Part model, mm, in its own coordinate system. A direction names the side the tool comes from. Give positions to 0.01 mm unless a question says otherwise; leave off trailing zeros. Order: outer loops, then holes, each group sorted by start corner. A loop starts at its lowest first (then second) coordinate and runs counter-clockwise, first axis right, second up. Notation, with made-up numbers: M 32.25,19.5 L 80.25,19.5 A18 cw 80.25,53.5 Z; hole C 2.25,32 d6. An arc over 180 degrees is marked long. One line per question, with ' | ' between items.
```python
from build123d import *

# Parameters (mm, degrees)
SKETCH_1_W          = 20
SKETCH_1_H          = 20
SKETCH_1_W_2        = 16
SKETCH_1_H_2        = 16
EXTRUDE_1_DEPTH     = 970
SKETCH_2_R          = 4.05
CUT_EXTRUDE_1_DEPTH = 20
SKETCH_4_W          = 21.376287738
SKETCH_4_H          = 29.089038522
CUT_EXTRUDE_3_DEPTH = 50
SKETCH_5_R          = 2.2
CUT_EXTRUDE_4_DEPTH = 30
SKETCH_6_R          = 1
CUT_EXTRUDE_5_DEPTH = 10
M4X0_7_1_D          = 3.3
M4X0_7_1_DEPTH      = 11.5
M4X0_7_1_TIP        = 0.991420021
SKETCH_12_R         = 1
CUT_EXTRUDE_7_DEPTH = 10
M4X0_7_6_D          = 3.3
M4X0_7_6_DEPTH      = 11.5
M4X0_7_6_TIP        = 0.991420021
SKETCH_15_R         = 2.1
CUT_EXTRUDE_8_DEPTH = 21
SKETCH_16_R         = 1
CUT_EXTRUDE_9_DEPTH = 10
M4X0_7_7_D          = 3.3
M4X0_7_7_DEPTH      = 11.5
M4X0_7_7_TIP        = 0.991420021


with BuildPart() as part:
    # ｽｹｯﾁ1 → ﾎﾞｽ - 押し出し1 (new body)
    with BuildSketch(Plane.XY):
        Rectangle(SKETCH_1_W, SKETCH_1_H)
        Rectangle(SKETCH_1_W_2, SKETCH_1_H_2, mode=Mode.SUBTRACT)
    extrude(amount=EXTRUDE_1_DEPTH)

    # ｽｹｯﾁ2 → ｶｯﾄ - 押し出し1 (cut)
    with BuildSketch(Plane(origin=(10, 0, 0), x_dir=(0, 0, -1), z_dir=(1, 0, 0))):
        with Locations((-50, 0)):
            Circle(SKETCH_2_R)
    extrude(amount=-CUT_EXTRUDE_1_DEPTH, mode=Mode.SUBTRACT)

    # ｽｹｯﾁ4 → ｶｯﾄ - 押し出し3 (cut)
    with BuildSketch(Plane.XY.offset(970)):
        Rectangle(SKETCH_4_W, SKETCH_4_H)
    extrude(amount=-CUT_EXTRUDE_3_DEPTH, mode=Mode.SUBTRACT)

    # ｽｹｯﾁ5 → ｶｯﾄ - 押し出し4 (cut)
    with BuildSketch(Plane(origin=(10, 0, 0), x_dir=(0, 0, -1), z_dir=(1, 0, 0))):
        with Locations((-816, 0)):
            Circle(SKETCH_5_R)
    extrude(amount=-CUT_EXTRUDE_4_DEPTH, mode=Mode.SUBTRACT)

    # ｽｹｯﾁ6 → ｶｯﾄ - 押し出し5 (cut)
    with BuildSketch(Plane.XZ.offset(10)):
        with Locations((0, 30)):
            Circle(SKETCH_6_R)
        with Locations((0, 50)):
            Circle(SKETCH_6_R)
    extrude(amount=-CUT_EXTRUDE_5_DEPTH, mode=Mode.SUBTRACT)

    # M4x0.7 ねじ穴1
    with Locations(Plane(origin=(0, -10, 30), x_dir=(0, 0, -1), z_dir=(0, -1, 0))):
        with Locations((0, 0), (-20, 0)):
            Hole(M4X0_7_1_D / 2, depth=M4X0_7_1_DEPTH)
            with Locations((0, 0, -(M4X0_7_1_DEPTH + M4X0_7_1_TIP / 2))):  # 118° drill point
                Cone(0, M4X0_7_1_D / 2, M4X0_7_1_TIP, mode=Mode.SUBTRACT)

    # ｽｹｯﾁ12 → ｶｯﾄ - 押し出し7 (cut)
    with BuildSketch(Plane(origin=(10, 0, 0), x_dir=(0, 0, -1), z_dir=(1, 0, 0))):
        with Locations((-40, 0)):
            Circle(SKETCH_12_R)
        with Locations((-710, 0)):
            Circle(SKETCH_12_R)
        with Locations((-730, 0)):
            Circle(SKETCH_12_R)
    extrude(amount=-CUT_EXTRUDE_7_DEPTH, mode=Mode.SUBTRACT)

    # M4x0.7 ねじ穴6
    with Locations(Plane(origin=(10, 0, 40), x_dir=(0, 0, 1), z_dir=(1, 0, 0))):
        with Locations((0, 0)):
            Hole(M4X0_7_6_D / 2, depth=M4X0_7_6_DEPTH)
            with Locations((0, 0, -(M4X0_7_6_DEPTH + M4X0_7_6_TIP / 2))):  # 118° drill point
                Cone(0, M4X0_7_6_D / 2, M4X0_7_6_TIP, mode=Mode.SUBTRACT)

    # ｽｹｯﾁ15 → ｶｯﾄ - 押し出し8 (cut, through all)
    with BuildSketch(Plane(origin=(10, 0, 0), x_dir=(0, 0, -1), z_dir=(1, 0, 0))):
        with Locations((-710, 0)):
            Circle(SKETCH_15_R)
        with Locations((-730, 0)):
            Circle(SKETCH_15_R)
    extrude(amount=-CUT_EXTRUDE_8_DEPTH, mode=Mode.SUBTRACT)

    # ｽｹｯﾁ16 → ｶｯﾄ - 押し出し9 (cut)
    with BuildSketch(Plane(origin=(0, -10, 0), x_dir=(-1, 0, 0), z_dir=(0, -1, 0))):
        with Locations((0, -670)):
            Circle(SKETCH_16_R)
        with Locations((0, -650)):
            Circle(SKETCH_16_R)
    extrude(amount=-CUT_EXTRUDE_9_DEPTH, mode=Mode.SUBTRACT)

    # M4x0.7 ねじ穴7
    with Locations(Plane(origin=(0, -10, 670), x_dir=(0, 0, -1), z_dir=(0, -1, 0))):
        with Locations((0, 0), (20, 0)):
            Hole(M4X0_7_7_D / 2, depth=M4X0_7_7_DEPTH)
            with Locations((0, 0, -(M4X0_7_7_DEPTH + M4X0_7_7_TIP / 2))):  # 118° drill point
                Cone(0, M4X0_7_7_D / 2, M4X0_7_7_TIP, mode=Mode.SUBTRACT)


solid = part.part
```
1. Probe L1, parallel to Z at x = -8.75, y = -0.5; L2, parallel to Y at x = 1, z = 246. List the from-to ranges inside material, lowest first. Write a range as from..to.
Worked out:
L1: z = 0..45.98, 54.02..707.96, 712.04..727.96, 732.04..813.86, 818.14..920 | L2: y = -10..-8, 8..10
2. Drop flat-ended pins along their axis: pin 1 (5.5 mm diameter, centred on y = 0, z = 730, fed in from +X); pin 2 (2 mm diameter, centred on x = 0, z = 50, fed in from -Y). Give the stop position or say it passes through.
Worked out:
pin 1: stops at x = 10 | pin 2: stops at y = 8
3. Slice it at A-A on z = 473. Give the cut face in (x, y), then the cut area to 3 significant figures.
Worked out:
outline: M -10,-10 L 10,-10 L 10,10 L -10,10 Z; hole M -8,-8 L 8,-8 L 8,8 L -8,8 Z | area: 144 mm2
4. Tool access for faces 1 (the flat face through (-10, 0, 454)), 2 (the flat face through (-8, 0, 454)): list every direction of +Z, -Z, +X, -X, +Y, -Y with a clear straight run to the whole face (end or side of a thin tool).
Worked out:
face 1: +Z, -Z, -X, +Y, -Y | face 2: +Z, -Z
5. Mould opens along Y. For faces 3 (the flat face through (-9, 0, 920)), 4 (the flat face through (0, -8, 454)), 5 (the flat face through (0, 10, 454)), 6 (the flat face through (0, 8, 454)) say: released by +Y, released by -Y, zero draft, split by the parting line, or undercut.
Worked out:
face 3: zero draft | face 4: undercut | face 5: released by +Y | face 6: undercut
